```python
from build123d import *

# Parameters (mm, degrees)
F1_DEPTH = 15
F4_W     = 17.5
F4_H     = 2.5
F5_DEPTH = 5.7


with BuildPart() as f1:
    # F0 (on Top) → F1 (new body)
    with BuildSketch(Plane.XY):
        with BuildLine():
            Line((0, 16.5), (0, 0))
            Line((0, 0), (-5.3, 0))
            Line((-5.3, 0), (-5.3, 16.5))
            ThreePointArc((-5.3, 16.5), (-5.592893, 17.207107), (-6.3, 17.5))
            ThreePointArc((-6.3, 17.5), (-9.128427, 16.328427), (-10.3, 13.5))
            Line((-10.3, 13.5), (-10.3, -3))
            ThreePointArc((-10.3, -3), (-9.714214, -4.414214), (-8.3, -5))
            Line((-8.3, -5), (-7.871245, -5))
            ThreePointArc((-7.871245, -5), (-1.868513, -6.468859), (2.777732, -10.543506))
            Line((2.777732, -10.543506), (14.339411, -27.055295))
            ThreePointArc((14.339411, -27.055295), (15.012235, -28.419648), (15.243651, -29.923177))
            Line((15.243651, -29.923177), (15.243651, -53.346683))
            Line((15.243651, -53.346683), (11.743651, -53.346683))
            ThreePointArc((11.743651, -53.346683), (10.682991, -53.786023), (10.243651, -54.846683))
            Line((10.243651, -54.846683), (10.243651, -55.846683))
            ThreePointArc((10.243651, -55.846683), (10.536544, -56.55379), (11.243651, -56.846683))
            Line((11.243651, -56.846683), (24.243651, -56.846683))
            ThreePointArc((24.243651, -56.846683), (24.950757, -56.55379), (25.243651, -55.846683))
            Line((25.243651, -55.846683), (25.243651, -54.846683))
            ThreePointArc((25.243651, -54.846683), (24.804311, -53.786023), (23.743651, -53.346683))
            Line((23.743651, -53.346683), (20.243651, -53.346683))
            Line((20.243651, -53.346683), (20.243651, -28.346683))
            ThreePointArc((20.243651, -28.346683), (20.012235, -26.843154), (19.339411, -25.478801))
            Line((19.339411, -25.478801), (5.90424, -6.291388))
            ThreePointArc((5.90424, -6.291388), (5.231415, -4.927035), (5, -3.423506))
            Line((5, -3.423506), (5, 13.5))
            ThreePointArc((5, 13.5), (3.828427, 16.328427), (1, 17.5))
            ThreePointArc((1, 17.5), (0.292893, 17.207107), (0, 16.5))
        make_face()
    extrude(amount=F1_DEPTH)


with BuildPart() as f2_1:
    # F2: instance of F1
    add(f1.part.mirror(Plane(origin=(-10.3, 5.25, 7.5), x_dir=(0, -1, 0), z_dir=(-1, 0, 0))))

    # F4 (on face) → F5 (cut)
    with BuildSketch(Plane.YZ.offset(-10.3)):
        with Locations((8.75, 13.75)):
            Rectangle(F4_W, F4_H)
    extrude(amount=-F5_DEPTH, mode=Mode.SUBTRACT)


solid = f2_1.part
```
Source: CAD feature listing. Evaluate the final solid. Frame: model axes, mm. A direction names the side the tool comes from. Coordinates: 2 decimals unless noted, no trailing zeros. Loops run counter-clockwise (first coordinate to the right, second up) from the corner with the lowest first, then second, coordinate; pieces in that order, holes last. Notation, with made-up numbers: M 47.25,-4 L 79.25,-4 A19 cw 79.25,6 Z; hole C -38.75,37.25 d6. An arc over 180 degrees is marked long. Use a Markdown table: item, result. Add a question column.
Q1. Section query D-D, the plane z = 9.5. Return loops of the section in (x, y).
Q2. Section query C-C, the plane x = -42. Return loops of the section in (y, z), and give its area (3 significant figures).
Q3. Draft query along X for faces 4 (the flat face through (-20.6, 8, 7)), 5 (the cylindrical face through (-24.459, 16.297, 7.395)), 6 (the flat face through (-35.844, -41, 7)), 7 (the flat face through (-13, 9, 12.5)). Return one class per face: pulls with the +X half, pulls with the -X half, needs draft (parallel to the pull), parting line crosses it, or undercut.
Q4. First-contact query: pin 1 (3 mm diameter, centred on x = -34, z = 10, fed in from +Y); pin 2 (7.5 mm diameter, centred on y = 1.5, z = 7, fed in from -X); pin 3 (1.5 mm diameter, centred on x = -11.5, y = 9, fed in from +Z); pin 4 (1 mm diameter, centred on x = -18.5, y = 7.5, fed in from +Z). Flat tips, straight axial feed; report the tip coordinate or a pass-through.
Q5. Section query A-A, the plane y = 10.5. Return loops of the section in (x, z), and give its area (4 significant figures).
Q6. Section query B-B, the plane z = 14.25. Return loops of the section in (x, y).
Q7. Access query for faces 1 (the flat face through (-34, -53.347, 7)), 2 (the flat face through (-15.3, 8, 6)), 3 (the flat face through (-40.844, -41, 7)). Directions: +Z, -Z, +X, -X, +Y, -Y. A direction counts if a zero-diameter tool reaches every point of the face in a straight line with its end or side. Return the directions, or none.
Q8. Material intervals for L1, parallel to X at y = 3.5, z = 7.5; L2, parallel to X at y = -31, z = 4.75; L3, parallel to X at y = -2.5, z = 4.5, sorted ascending.
Result:
| question | item | result |
|---|---|---|
| 1 | outline | M -45.84,-55.85 A1 ccw -44.84,-56.85 L -31.84,-56.85 A1 ccw -30.84,-55.85 L -30.84,-54.85 A1.5 ccw -32.34,-53.35 L -35.84,-53.35 L -35.84,-29.92 A5 cw -34.94,-27.06 L -23.38,-10.54 A13 cw -12.73,-5 L -12.3,-5 A2 ccw -10.3,-3 L -10.3,13.5 A4 ccw -14.3,17.5 A1 ccw -15.3,16.5 L -15.3,0 L -20.6,0 L -20.6,16.5 A1 ccw -21.6,17.5 A4 ccw -25.6,13.5 L -25.6,-3.42 A5 cw -26.5,-6.29 L -39.94,-25.48 A5 ccw -40.84,-28.35 L -40.84,-53.35 L -44.34,-53.35 A1.5 ccw -45.84,-54.85 Z |
| 2 | outline | M -56.85,0 L -53.35,0 L -53.35,15 L -56.85,15 Z |
| 2 | area | 52.5 mm2 |
| 3 | face 4 | undercut |
| 3 | face 5 | pulls with the -X half |
| 3 | face 6 | pulls with the +X half |
| 3 | face 7 | needs draft |
| 4 | pin 1 | stops at y = -14.85 |
| 4 | pin 2 | stops at x = -25.6 |
| 4 | pin 3 | stops at z = 12.5 |
| 4 | pin 4 | passes through |
| 5 | outline | M -25.6,0 L -20.6,0 L -20.6,15 L -25.6,15 Z; M -15.3,0 L -10.3,0 L -10.3,12.5 L -15.3,12.5 Z |
| 5 | area | 137.5 mm2 |
| 6 | outline | M -45.84,-55.85 A1 ccw -44.84,-56.85 L -31.84,-56.85 A1 ccw -30.84,-55.85 L -30.84,-54.85 A1.5 ccw -32.34,-53.35 L -35.84,-53.35 L -35.84,-29.92 A5 cw -34.94,-27.06 L -23.38,-10.54 A13 cw -12.73,-5 L -12.3,-5 A2 ccw -10.3,-3 L -10.3,0 L -20.6,0 L -20.6,16.5 A1 ccw -21.6,17.5 A4 ccw -25.6,13.5 L -25.6,-3.42 A5 cw -26.5,-6.29 L -39.94,-25.48 A5 ccw -40.84,-28.35 L -40.84,-53.35 L -44.34,-53.35 A1.5 ccw -45.84,-54.85 Z |
| 7 | face 1 | +Z, -Z, +X |
| 7 | face 2 | +Z, -Z, +Y |
| 7 | face 3 | +Z, -Z, -X, +Y |
| 8 | L1 | x = -25.6 to -20.6, -15.3 to -10.3 |
| 8 | L2 | x = -40.84 to -35.84 |
| 8 | L3 | x = -25.6 to -10.3 |
